Answer from the drawing. Dimensions are ordinates in mm from the lowest x, y and z of the part. A direction names the side the tool comes from. Give positions to 0.01 mm unless a question says otherwise; leave off trailing zeros. Loops run counter-clockwise (first coordinate to the right, second up) from the corner with the lowest first, then second, coordinate; pieces in that order, holes last. Notation, with made-up numbers: (54.5, 69.25) -> (102.5, 69.25) arc R16 ccw to (102.5, 88.25) -> close; hole circle Ø8 at (81, -33.5). An arc over 180 degrees is marked (long way). Write each question's results on one line, items separated by ' | '. Start each with the question number.
Item 1: Determine the mould class of the marked faces 1, 2 and 3 for opening direction X: +X half, -X half, draft (parallel to the pull), parting line (faces both ways), or undercut.
Item 2: Find the intervals of material crossed by line 1 (Y direction, x = 7, z = 15); line 2 (Y direction, x = 7.75, z = 12) (1 decimal); line 3 (Z direction, x = 7.5, y = 3.5), in increasing order.
Item 3: Each of these flat-tipped pins is pushed along its axis until it touches: P1, Ø4, axis at y = 9, z = 11.5, coming from the -X side; P2, Ø6, axis at x = 2, z = 8, coming from the -Y side; P3, Ø1.5, axis at x = 3, z = 9.5, coming from the +Y side; P4, Ø2.5, axis at x = 5.5, y = 6.5, coming from the -Z side. Where does it stop, or does it pass through?
Item 4: Section A-A on x = 7 is taken. Write down the section's boundary in (y, z).
Item 5: Section B-B on z = 6 is taken. Write down the section's boundary in (x, y).
Item 6: Section C-C on y = 8 is taken. Write down the section's boundary in (x, z).
Item 7: Section D-D on x = 2.75 is taken. Write down the section's boundary in (y, z), and give its area (3 significant figures).
Item 8: Which of the six approach directions +Z, -Z, +X, -X, +Y, -Y give full straight-line access (tool end or side, diameter ignored) to the marked faces 4 and 5?
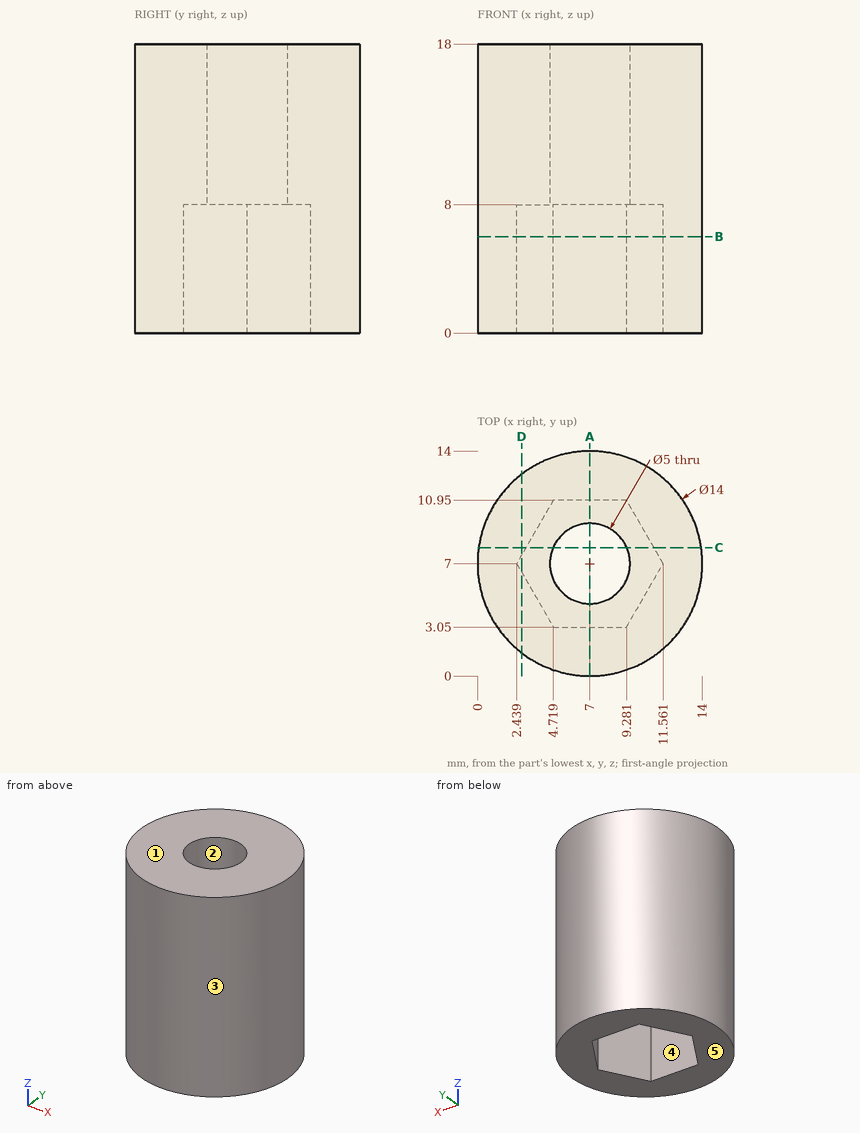
Findings:
1) face 1: draft | face 2: undercut | face 3: parting line
2) line 1: 0 to 4.5, 9.5 to 14 | line 2: 0 to 4.6, 9.4 to 14 | line 3: 8 to 18
3) P1: x = 0 | P2: y = 0.29 | P3: y = 13.2 | P4: z = 8
4) outline: (0, 0) -> (3.05, 0) -> (3.05, 8) -> (4.5, 8) -> (4.5, 18) -> (0, 18) -> close; (9.5, 8) -> (10.95, 8) -> (10.95, 0) -> (14, 0) -> (14, 18) -> (9.5, 18) -> close
5) outline: circle Ø14 at (7, 7); hole (2.44, 7) -> (4.72, 3.05) -> (9.28, 3.05) -> (11.56, 7) -> (9.28, 10.95) -> (4.72, 10.95) -> close
6) outline: (0.07, 0) -> (3.02, 0) -> (3.02, 8) -> (4.71, 8) -> (4.71, 18) -> (0.07, 18) -> close; (9.29, 8) -> (10.98, 8) -> (10.98, 0) -> (13.93, 0) -> (13.93, 18) -> (9.29, 18) -> close
7) outline: (1.44, 0) -> (6.46, 0) -> (6.46, 8) -> (7.54, 8) -> (7.54, 0) -> (12.56, 0) -> (12.56, 18) -> (1.44, 18) -> close | area: 192 mm2
8) face 4: -Z | face 5: -Z, +X, -X, +Y, -Y
